from build123d import *
from build123d import SkipClean  # not in build123d's __all__

# Parameters (mm, degrees)
F1_ANGLE_BACK = 90
F1_ANGLE      = 180
F2_ANGLE_BACK = 90
F2_ANGLE      = 180
F3_DEPTH      = 5.5
F4_R          = 0.5


with BuildPart() as f1:
    # F0 (on Top) → F1 (revolve)
    with BuildSketch(Plane.XY, mode=Mode.PRIVATE) as f1_sk:
        Polygon((23, 0), (0, 0), (0, -1.5), (0, -3.75), (21.5, -3.75), (21.5, -5.25), (23, -5.25), (23, -3.75), (23, -1.5), align=None)
        Polygon((0, -3.75), (0, -1.5), (-11.5, -1.5), (-23, -1.5), (-26.75, -1.5), (-23, -5.25), (-23, -3.75), align=None)
    revolve(f1_sk.sketch.rotate(Axis((11.5, 0, 0), (1, 0, 0)), -F1_ANGLE_BACK), axis=Axis((11.5, 0, 0), (1, 0, 0)), revolution_arc=F1_ANGLE)

    # F0 (on Top) → F2 (revolve)
    with BuildSketch(Plane.XY, mode=Mode.PRIVATE) as f2_sk:
        Polygon((21.5, 5.25), (21.5, 3.75), (11.5, 3.75), (0, 3.75), (0, 1.5), (0, 0), (23, 0), (23, 1.5), (23, 3.75), (23, 5.25), align=None)
        Polygon((0, 1.5), (0, 3.75), (-23, 3.75), (-23, 5.25), (-26.75, 1.5), (-23, 1.5), (-11.5, 1.5), align=None)
    revolve(f2_sk.sketch.rotate(Axis((11.5, 0, 0), (1, 0, 0)), -F2_ANGLE_BACK), axis=Axis((11.5, 0, 0), (1, 0, 0)), revolution_arc=F2_ANGLE)

    # F0 (on Top) → F3 (cut, symmetric)
    with BuildSketch(Plane.XY):
        Polygon((0, 0), (0, 1.5), (-11.5, 1.5), (-23, 1.5), (-26.75, 1.5), (-26.75, -1.5), (-23, -1.5), (-11.5, -1.5), (0, -1.5), align=None)
    with SkipClean():  # cleaning this boolean's faces spoils the solid; the shape is the same uncleaned
        extrude(amount=F3_DEPTH, both=True, mode=Mode.SUBTRACT)

    # F4
    f4_edges = [f1.edges().sort_by_distance(p)[0] for p in [
        (-23, 3.75, 0),
        (-23, -3.75, 0),
    ]]
    fillet(f4_edges, radius=F4_R)


solid = f1.part
Geometry check sheet. Reference: the model listing, model coordinates, mm. A direction names the side the tool comes from. Give positions to 0.01 mm unless a question says otherwise; leave off trailing zeros. Order: outer loops, then holes, each group sorted by start corner. A loop starts at its lowest first (then second) coordinate and runs counter-clockwise, first axis right, second up.
1. Sectioned sample at B-B (y = 0). Record the boundary of the cut face in (x, z).
Completed:
outline: (0, -3.75) - (21.5, -3.75) - (21.5, -5.25) - (23, -5.25) - (23, 5.25) - (21.5, 5.25) - (21.5, 3.75) - (0, 3.75) - close
2. Sectioned sample at A-A (z = 0). Record the boundary of the cut face in (x, y).
Completed:
outline: (-26.75, -1.5) - (-23, -5.25) - (-23, -4.25) arc R0.5 cw to (-22.5, -3.75) - (21.5, -3.75) - (21.5, -5.25) - (23, -5.25) - (23, 5.25) - (21.5, 5.25) - (21.5, 3.75) - (-22.5, 3.75) arc R0.5 cw to (-23, 4.25) - (-23, 5.25) - (-26.75, 1.5) - (0, 1.5) - (0, -1.5) - close
3. Sectioned sample at C-C (x = -13.5). Record the boundary of the cut face in (y, z).
Completed:
outline: (-1.5, -3.44) - (-1.5, 3.44) arc R3.75 ccw to start; (1.5, -3.44) arc R3.75 ccw to (1.5, 3.44) - close
4. Scan lines: line 1 (Y direction, x = 7, z = 0.25); line 2 (X direction, y = 5, z = -0.25); line 3 (Y direction, x = -14, z = -3). Record each from-to range of solid material in increasing order.
Completed:
line 1: y = -3.74 to 3.74
line 2: x = -23.24 to -23, 21.5 to 23
line 3: y = -2.25 to -1.5, 1.5 to 2.25
5. Depth check by flat-ended pin: pin 1 (6 mm diameter, centred on x = 1.5, z = -4, fed in from +Y); pin 2 (5 mm diameter, centred on y = 0, z = 1, fed in from -X); pin 3 (4 mm diameter, centred on x = -8, z = -0.5, fed in from +Y); pin 4 (1.5 mm diameter, centred on y = -0.5, z = 0.5, fed in from -X). Enter the tip coordinate at first touch or a pass-through.
Completed:
pin 1: stops at y = 3.61
pin 2: stops at x = -26.75
pin 3: stops at y = 3.75
pin 4: stops at x = 0
6. Access from +Z, -Z, +X, -X, +Y, -Y to the whole of each face (thin tool, end or side, straight path). Record for faces 5 (the face through (23, 0, 0)), 6 (the face through (-13, 1.5, 0)), 7 (the face through (-24.85, -3.4, 0.06)), 8 (the face through (-23, 4.4, 0)), 9 (the face through (-23, -4.4, 0)).
Completed:
face 5: +Z, -Z, +X, +Y, -Y
face 6: +Z, -Z, -X
face 7: -X, -Y
face 8: +Y
face 9: -Y
7. Draft check along X on faces 1 (the face through (21.5, 1, 4)), 2 (the face through (-0.808, -2.282, 2.976)), 3 (the face through (-14, -1.5, 0)), 4 (the face through (-24.9, 3.35, -0.06)). Enter one of: pulls with the +X half, pulls with the -X half, needs draft (parallel to the pull), parting line crosses it, or undercut.
Completed:
face 1: undercut
face 2: undercut
face 3: needs draft
face 4: pulls with the -X half
